Drawing for the job (mm, zero at the part's lowest x, y, z). A direction names the side the tool comes from. Round coordinates to 2 decimals unless told otherwise and drop trailing zeros. Order: outer loops, then holes, each group sorted by start corner. A loop starts at its lowest first (then second) coordinate and runs counter-clockwise, first axis right, second up. Notation, with made-up numbers: (-32.75, 44) -> (-19.75, 44) arc R18 cw to (-19.75, 59) -> close; hole circle Ø9 at (81.5, 85). An arc over 180 degrees is marked (long way). Use CSV: the item, a comma, the result in double quotes.
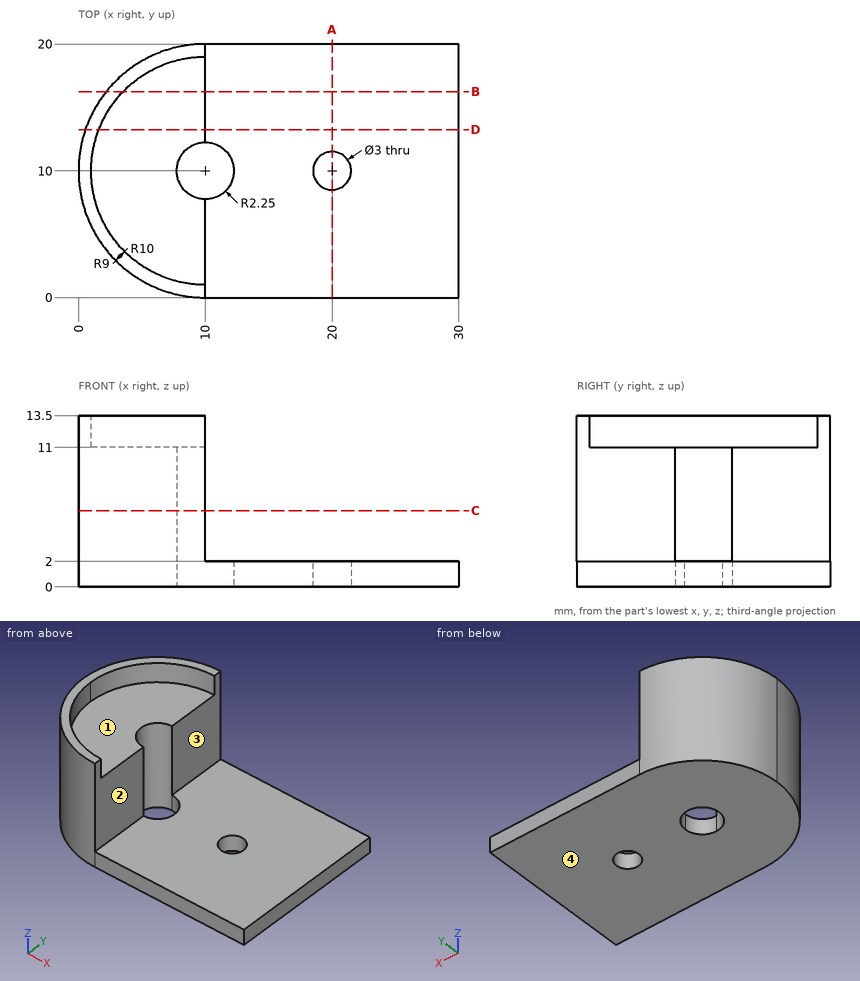
Q1. Cut at A-A (x = 20). Give the cut face in (y, z).
From the geometry:
outline,"(0, 0) -> (8.5, 0) -> (8.5, 2) -> (0, 2) -> close; (11.5, 0) -> (20, 0) -> (20, 2) -> (11.5, 2) -> close"
Q2. Cut at B-B (y = 16.25). Give the cut face in (x, z), plus the area to 3 significant figures.
From the geometry:
outline,"(2.19, 0) -> (30, 0) -> (30, 2) -> (10, 2) -> (10, 11) -> (3.52, 11) -> (3.52, 13.5) -> (2.19, 13.5) -> close"
area,"129 mm²"
Q3. Pin check, flat tips, straight feed: pin 1 (2.5 mm diameter, centred on x = 6, y = 12, fed in from +Z); pin 2 (4 mm diameter, centred on y = 18, z = 6.5, fed in from +X); pin 3 (10 mm diameter, centred on x = 21.5, y = 5.5, fed in from +Z). Stop position of each tip, or through.
From the geometry:
pin 1,"stops at z = 11"
pin 2,"stops at x = 10"
pin 3,"stops at z = 2"
Q4. Mould opens along Y. For the marked faces 1 and 2 say: +Y half, -Y half, draft (parallel to the pull), parting line (faces both ways), or undercut.
From the geometry:
face 1,"undercut"
face 2,"draft"
Q5. Probe line 1 along X through (y, z) = (9.5, 1.25); line 2 along Y through (x, z) = (20, 1.15); line 3 along Z through (x, y) = (23, 15.75). List the from-to ranges inside material, lowest first.
From the geometry:
line 1,"x = 0.01 to 7.81, 12.19 to 18.59, 21.41 to 30"
line 2,"y = 0 to 8.5, 11.5 to 20"
line 3,"z = 0 to 2"
Q6. Cut at C-C (z = 6). Give the cut face in (x, y).
From the geometry:
outline,"(0, 10) arc R10 ccw to (10, 0) -> (10, 7.75) arc R2.25 cw to (10, 12.25) -> (10, 20) arc R10 ccw to start"
Q7. Cut at D-D (y = 13.25). Give the cut face in (x, z), plus the area to 3 significant figures.
From the geometry:
outline,"(0.54, 0) -> (30, 0) -> (30, 2) -> (10, 2) -> (10, 11) -> (1.61, 11) -> (1.61, 13.5) -> (0.54, 13.5) -> close"
area,"147 mm²"
Q8. Which spindle directions (+Z, -Z, +X, -X, +Y, -Y) get a long thin tool onto all of the face, cutting with end or side? Do the marked faces 3 and 4. Say none if no direction does.
From the geometry:
face 3,"+Z, +X, +Y, -Y"
face 4,"-Z, +X, -X, +Y, -Y"
